For this review, use the dimensioned drawing (mm, ordinates from the lowest corner) and the shaded views. A direction names the side the tool comes from. Round coordinates to 2 decimals unless told otherwise and drop trailing zeros. Write each loop counter-clockwise with the first axis right and the second up, starting at its lowest first coordinate (ties: lowest second). Pieces come first, ordered by that corner, then holes. Notation, with made-up numbers: (85.5, 83.25) -> (92.5, 83.25) arc R24 ccw to (92.5, 121.25) -> close; hole circle Ø7 at (12, -36.5). An arc over 180 degrees is marked (long way). Write each question's results on one line, items separated by ' | '. Start each with the question number.
Item 1: To check wall thickness, follow line 1 along X through (y, z) = (21, 1); line 2 along Z through (x, y) = (48.5, 69.5); line 3 along Y through (x, z) = (100, 106.35). State the ranges of each line that lie inside material, in increasing order.
Item 2: Add section A-A (x = 375). State the section outline as (y, z) points, plus the area to 3 significant figures.
Item 3: Clearance check with flat-ended pins moving along their axes: pin 1 (4.5 mm diameter, centred on x = 100, y = 24.05, fed in from +Z); pin 2 (6 mm diameter, centred on x = 61.5, z = 41.5, fed in from +Y). State where each tip first meets the part, or that it passes through.
Item 4: Add section D-D (x = 132). State the section outline as (y, z) points.
Item 5: Tool access review of the marked faces 1 and 2: name each direction out of +Z, -Z, +X, -X, +Y, -Y from which nothing blocks a thin tool from reaching the whole face with its end or side.
Item 6: The part is to be moulded in two halves that separate along Z. For the marked faces 3, 4 and 5, say which applies: +Z half, -Z half, draft (parallel to the pull), parting line (faces both ways), or undercut.
Item 7: Add section B-B (y = 102.5). State the section outline as (x, z) points.
Item 8: Add section C-C (y = 84). State the section outline as (x, z) points, plus the area to 3 significant figures.
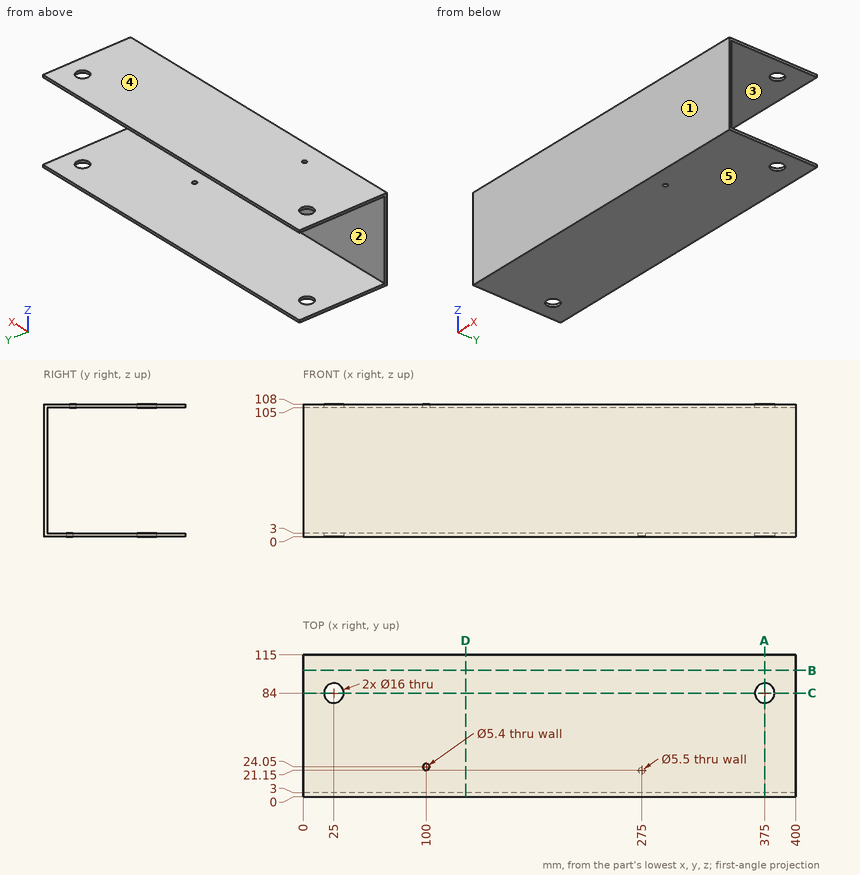
Responses:
1) line 1: x = 0 to 272.25, 277.75 to 400 | line 2: z = 0 to 3, 105 to 108 | line 3: y = 0 to 21.35, 26.75 to 115
2) outline: (0, 0) -> (76, 0) -> (76, 3) -> (3, 3) -> (3, 105) -> (76, 105) -> (76, 108) -> (0, 108) -> close; (92, 0) -> (115, 0) -> (115, 3) -> (92, 3) -> close; (92, 105) -> (115, 105) -> (115, 108) -> (92, 108) -> close | area: 900 mm^2
3) pin 1: stops at z = 3 | pin 2: stops at y = 3
4) outline: (0, 0) -> (115, 0) -> (115, 3) -> (3, 3) -> (3, 105) -> (115, 105) -> (115, 108) -> (0, 108) -> close
5) face 1: +Z, -Z, +X, -X, -Y | face 2: +X, -X, +Y
6) face 3: undercut | face 4: +Z half | face 5: -Z half
7) outline: (0, 0) -> (400, 0) -> (400, 3) -> (0, 3) -> close; (0, 105) -> (400, 105) -> (400, 108) -> (0, 108) -> close
8) outline: (0, 0) -> (17, 0) -> (17, 3) -> (0, 3) -> close; (0, 105) -> (17, 105) -> (17, 108) -> (0, 108) -> close; (33, 0) -> (367, 0) -> (367, 3) -> (33, 3) -> close; (33, 105) -> (367, 105) -> (367, 108) -> (33, 108) -> close; (383, 0) -> (400, 0) -> (400, 3) -> (383, 3) -> close; (383, 105) -> (400, 105) -> (400, 108) -> (383, 108) -> close | area: 2,210 mm^2
